```python
from build123d import *

# Parameters (mm, degrees)
RESSALTO_EXTRUS_O2_DEPTH = 9.2
ESBO_O5_R                = 2.15
CORTE_EXTRUS_O2_DEPTH    = 9.2
CHANFRO2_SIZE            = 0.3
SKETCH1_W                = 12.014068267
SKETCH1_H                = 17.223276929
CUT_EXTRUDE1_DEPTH       = 25
SKETCH3_W                = 4
SKETCH3_H                = 9.2
BOSS_EXTRUDE1_DEPTH      = 5
SKETCH4_R                = 1.5
CUT_EXTRUDE3_DEPTH       = 10
SKETCH5_W                = 42.60578415
SKETCH5_H                = 33.509789151
CUT_EXTRUDE4_DEPTH       = 1.1
SKETCH6_W                = 58.176505701
SKETCH6_H                = 25.888094607
CUT_EXTRUDE5_DEPTH       = 1.1
SKETCH7_W                = 20
SKETCH7_H                = 4.9
BOSS_EXTRUDE2_DEPTH      = 1.1
SKETCH8_W                = 20
SKETCH8_H                = 4.9
BOSS_EXTRUDE3_DEPTH      = 1.1


with BuildPart() as part:
    # Esboço4 → Ressalto-extrusão2 (new body)
    with BuildSketch(Plane(origin=(0, 0, 0), x_dir=(1, 0, 0), z_dir=(0, 1, 0))):
        with BuildLine():
            Line((-19.2, 2.35), (-19.2, 1.65))
            ThreePointArc((-19.2, 1.65), (-19.170710678, 1.579289322), (-19.1, 1.55))
            Line((-19.1, 1.55), (-18.1, 1.55))
            ThreePointArc((-18.1, 1.55), (-18.029289322, 1.579289322), (-18, 1.65))
            Line((-18, 1.65), (-18, 2.35))
            ThreePointArc((-18, 2.35), (-17.970710678, 2.420710678), (-17.9, 2.45))
            Line((-17.9, 2.45), (-17.3, 2.45))
            ThreePointArc((-17.3, 2.45), (-17.229289322, 2.420710678), (-17.2, 2.35))
            Line((-17.2, 2.35), (-17.2, 1.65))
            ThreePointArc((-17.2, 1.65), (-17.170710678, 1.579289322), (-17.1, 1.55))
            Line((-17.1, 1.55), (-16.1, 1.55))
            ThreePointArc((-16.1, 1.55), (-16.029289322, 1.579289322), (-16, 1.65))
            Line((-16, 1.65), (-16, 2.35))
            ThreePointArc((-16, 2.35), (-15.970710678, 2.420710678), (-15.9, 2.45))
            Line((-15.9, 2.45), (-15.3, 2.45))
            ThreePointArc((-15.3, 2.45), (-15.229289322, 2.420710678), (-15.2, 2.35))
            Line((-15.2, 2.35), (-15.2, 1.65))
            ThreePointArc((-15.2, 1.65), (-15.170710678, 1.579289322), (-15.1, 1.55))
            Line((-15.1, 1.55), (-14.1, 1.55))
            ThreePointArc((-14.1, 1.55), (-14.029289322, 1.579289322), (-14, 1.65))
            Line((-14, 1.65), (-14, 2.35))
            ThreePointArc((-14, 2.35), (-13.970710678, 2.420710678), (-13.9, 2.45))
            Line((-13.9, 2.45), (-13.3, 2.45))
            ThreePointArc((-13.3, 2.45), (-13.229289322, 2.420710678), (-13.2, 2.35))
            Line((-13.2, 2.35), (-13.2, 1.65))
            ThreePointArc((-13.2, 1.65), (-13.170710678, 1.579289322), (-13.1, 1.55))
            Line((-13.1, 1.55), (-12.1, 1.55))
            ThreePointArc((-12.1, 1.55), (-12.029289322, 1.579289322), (-12, 1.65))
            Line((-12, 1.65), (-12, 2.35))
            ThreePointArc((-12, 2.35), (-11.970710678, 2.420710678), (-11.9, 2.45))
            Line((-11.9, 2.45), (-11.3, 2.45))
            ThreePointArc((-11.3, 2.45), (-11.229289322, 2.420710678), (-11.2, 2.35))
            Line((-11.2, 2.35), (-11.2, 1.65))
            ThreePointArc((-11.2, 1.65), (-11.170710678, 1.579289322), (-11.1, 1.55))
            Line((-11.1, 1.55), (-10.1, 1.55))
            ThreePointArc((-10.1, 1.55), (-10.029289322, 1.579289322), (-10, 1.65))
            Line((-10, 1.65), (-10, 2.35))
            ThreePointArc((-10, 2.35), (-9.970710678, 2.420710678), (-9.9, 2.45))
            Line((-9.9, 2.45), (-9.3, 2.45))
            ThreePointArc((-9.3, 2.45), (-9.229289322, 2.420710678), (-9.2, 2.35))
            Line((-9.2, 2.35), (-9.2, 1.65))
            ThreePointArc((-9.2, 1.65), (-9.170710678, 1.579289322), (-9.1, 1.55))
            Line((-9.1, 1.55), (-8.1, 1.55))
            ThreePointArc((-8.1, 1.55), (-8.029289322, 1.579289322), (-8, 1.65))
            Line((-8, 1.65), (-8, 2.35))
            ThreePointArc((-8, 2.35), (-7.970710678, 2.420710678), (-7.9, 2.45))
            Line((-7.9, 2.45), (-7.3, 2.45))
            ThreePointArc((-7.3, 2.45), (-7.229289322, 2.420710678), (-7.2, 2.35))
            Line((-7.2, 2.35), (-7.2, 1.65))
            ThreePointArc((-7.2, 1.65), (-7.170710678, 1.579289322), (-7.1, 1.55))
            Line((-7.1, 1.55), (7.1, 1.55))
            ThreePointArc((7.1, 1.55), (7.170710678, 1.579289322), (7.2, 1.65))
            Line((7.2, 1.65), (7.2, 2.35))
            ThreePointArc((7.2, 2.35), (7.229289322, 2.420710678), (7.3, 2.45))
            Line((7.3, 2.45), (7.9, 2.45))
            ThreePointArc((7.9, 2.45), (7.970710678, 2.420710678), (8, 2.35))
            Line((8, 2.35), (8, 1.65))
            ThreePointArc((8, 1.65), (8.029289322, 1.579289322), (8.1, 1.55))
            Line((8.1, 1.55), (9.1, 1.55))
            ThreePointArc((9.1, 1.55), (9.170710678, 1.579289322), (9.2, 1.65))
            Line((9.2, 1.65), (9.2, 2.35))
            ThreePointArc((9.2, 2.35), (9.229289322, 2.420710678), (9.3, 2.45))
            Line((9.3, 2.45), (9.9, 2.45))
            ThreePointArc((9.9, 2.45), (9.970710678, 2.420710678), (10, 2.35))
            Line((10, 2.35), (10, 1.65))
            ThreePointArc((10, 1.65), (10.029289322, 1.579289322), (10.1, 1.55))
            Line((10.1, 1.55), (11.1, 1.55))
            ThreePointArc((11.1, 1.55), (11.170710678, 1.579289322), (11.2, 1.65))
            Line((11.2, 1.65), (11.2, 2.35))
            ThreePointArc((11.2, 2.35), (11.229289322, 2.420710678), (11.3, 2.45))
            Line((11.3, 2.45), (11.9, 2.45))
            ThreePointArc((11.9, 2.45), (11.970710678, 2.420710678), (12, 2.35))
            Line((12, 2.35), (12, 1.65))
            ThreePointArc((12, 1.65), (12.029289322, 1.579289322), (12.1, 1.55))
            Line((12.1, 1.55), (13.1, 1.55))
            ThreePointArc((13.1, 1.55), (13.170710678, 1.579289322), (13.2, 1.65))
            Line((13.2, 1.65), (13.2, 2.35))
            ThreePointArc((13.2, 2.35), (13.229289322, 2.420710678), (13.3, 2.45))
            Line((13.3, 2.45), (13.9, 2.45))
            ThreePointArc((13.9, 2.45), (13.970710678, 2.420710678), (14, 2.35))
            Line((14, 2.35), (14, 1.65))
            ThreePointArc((14, 1.65), (14.029289322, 1.579289322), (14.1, 1.55))
            Line((14.1, 1.55), (15.1, 1.55))
            ThreePointArc((15.1, 1.55), (15.170710678, 1.579289322), (15.2, 1.65))
            Line((15.2, 1.65), (15.2, 2.35))
            ThreePointArc((15.2, 2.35), (15.229289322, 2.420710678), (15.3, 2.45))
            Line((15.3, 2.45), (15.9, 2.45))
            ThreePointArc((15.9, 2.45), (15.970710678, 2.420710678), (16, 2.35))
            Line((16, 2.35), (16, 1.65))
            ThreePointArc((16, 1.65), (16.029289322, 1.579289322), (16.1, 1.55))
            Line((16.1, 1.55), (17.1, 1.55))
            ThreePointArc((17.1, 1.55), (17.170710678, 1.579289322), (17.2, 1.65))
            Line((17.2, 1.65), (17.2, 2.35))
            ThreePointArc((17.2, 2.35), (17.229289322, 2.420710678), (17.3, 2.45))
            Line((17.3, 2.45), (17.9, 2.45))
            ThreePointArc((17.9, 2.45), (17.970710678, 2.420710678), (18, 2.35))
            Line((18, 2.35), (18, 1.65))
            ThreePointArc((18, 1.65), (18.029289322, 1.579289322), (18.1, 1.55))
            Line((18.1, 1.55), (19.1, 1.55))
            ThreePointArc((19.1, 1.55), (19.170710678, 1.579289322), (19.2, 1.65))
            Line((19.2, 1.65), (19.2, 2.35))
            ThreePointArc((19.2, 2.35), (19.229289322, 2.420710678), (19.3, 2.45))
            Line((19.3, 2.45), (19.9, 2.45))
            ThreePointArc((19.9, 2.45), (19.970710678, 2.420710678), (20, 2.35))
            Line((20, 2.35), (20, -2.45))
            Line((20, -2.45), (-20, -2.45))
            Line((-20, -2.45), (-20, 2.35))
            ThreePointArc((-20, 2.35), (-19.970710678, 2.420710678), (-19.9, 2.45))
            Line((-19.9, 2.45), (-19.3, 2.45))
            ThreePointArc((-19.3, 2.45), (-19.229289322, 2.420710678), (-19.2, 2.35))
        make_face()
    extrude(amount=RESSALTO_EXTRUS_O2_DEPTH)

    # Esboço5 → Corte-extrusão2 (cut)
    with BuildSketch(Plane(origin=(0, 0, -1.55), x_dir=(-1, 0, 0), z_dir=(0, 0, -1))):
        with Locations((0, 4.6)):
            Circle(ESBO_O5_R)
    extrude(amount=-CORTE_EXTRUS_O2_DEPTH, mode=Mode.SUBTRACT)

    # Chanfro2
    chanfro2_edges = [part.edges().sort_by_distance(p)[0] for p in [
        (2.15, 4.6, -1.55),
    ]]
    chamfer(chanfro2_edges, length=CHANFRO2_SIZE)

    # Sketch1 → Cut-Extrude1 (cut)
    with BuildSketch(Plane(origin=(20, 0, 0), x_dir=(0, 0, -1), z_dir=(1, 0, 0))):
        with Locations((-0.254525551, 3.53223116)):
            Rectangle(SKETCH1_W, SKETCH1_H)
    extrude(amount=-CUT_EXTRUDE1_DEPTH, mode=Mode.SUBTRACT)

    # Sketch3 → Boss-Extrude1 (add)
    with BuildSketch(Plane(origin=(-5, 0, 0), x_dir=(0, 0, -1), z_dir=(1, 0, 0))):
        with Locations((-0.45, 4.6)):
            Rectangle(SKETCH3_W, SKETCH3_H)
    extrude(amount=BOSS_EXTRUDE1_DEPTH)

    # Sketch4 → Cut-Extrude3 (cut)
    with BuildSketch(Plane(origin=(0, 0, -1.55), x_dir=(-1, 0, 0), z_dir=(0, 0, -1))):
        with Locations((5, 4.6)):
            Circle(SKETCH4_R)
    extrude(amount=-CUT_EXTRUDE3_DEPTH, mode=Mode.SUBTRACT)

    # Sketch5 → Cut-Extrude4 (cut)
    with BuildSketch(Plane.XZ):
        with Locations((-12.27909741, -6.492410197)):
            Rectangle(SKETCH5_W, SKETCH5_H)
    extrude(amount=-CUT_EXTRUDE4_DEPTH, mode=Mode.SUBTRACT)

    # Sketch6 → Cut-Extrude5 (cut)
    with BuildSketch(Plane(origin=(0, 9.2, 0), x_dir=(1, 0, 0), z_dir=(0, 1, 0))):
        with Locations((-5.279993837, 3.701095613)):
            Rectangle(SKETCH6_W, SKETCH6_H)
    extrude(amount=-CUT_EXTRUDE5_DEPTH, mode=Mode.SUBTRACT)

    # Sketch7 → Boss-Extrude2 (add)
    with BuildSketch(Plane(origin=(0, 8.1, 0), x_dir=(1, 0, 0), z_dir=(0, 1, 0))):
        with Locations((-10, 0)):
            Rectangle(SKETCH7_W, SKETCH7_H)
    extrude(amount=BOSS_EXTRUDE2_DEPTH)

    # Sketch8 → Boss-Extrude3 (add)
    with BuildSketch(Plane.XZ.offset(-1.1)):
        with Locations((-10, 0)):
            Rectangle(SKETCH8_W, SKETCH8_H)
    extrude(amount=BOSS_EXTRUDE3_DEPTH)


solid = part.part
```
Model file for the job. Use its own axes, mm. A direction names the side the tool comes from. Give positions to 0.01 mm unless a question says otherwise; leave off trailing zeros. Loops run counter-clockwise (first coordinate to the right, second up) from the corner with the lowest first, then second, coordinate; pieces in that order, holes last. Notation, with made-up numbers: (-31.5, 43.25) - (-24.5, 43.25) arc R23 cw to (-24.5, 57.25) - close; hole circle Ø2 at (31.25, 47). An arc over 180 degrees is marked (long way). One line per item, written item: value. Start each with the question number.
1. Pin check, flat tips, straight feed: pin 1 (3.5 mm diameter, centred on x = -5, y = 6, fed in from -Z); pin 2 (1.1 mm diameter, centred on x = -15, y = 3.5, fed in from -Z). Stop position of each tip, or through.
2. Slice it at C-C (z = 0.3). List the corners of the cut face in (x, y).
3. Pull direction Y, two halves, no side cores. Call faces 1 (the flat face through (-15, 8.1, -2)), 2 (the flat face through (-10, 9.2, 0)), 3 (the flat face through (0, 5, 1)): pulls with the +Y half, pulls with the -Y half, needs draft (parallel to the pull), parting line crosses it, or undercut.
4. Slice it at A-A (x = -5). List the corners of the cut face in (y, z), plus the area to 3 significant figures.
5. Slice it at B-B (z = -2). Give the number of separate pieces and of enclosed holes in the cut face, plus the area to 3 significant figures.
6. Probe L1, parallel to Y at x = -5, z = -0.4; L2, parallel to Y at x = -16.75, z = -2.15; L3, parallel to Z at x = -1.75, y = 7. List the from-to ranges inside material, lowest first. Write a range as from..to.
7. Which spindle directions (+Z, -Z, +X, -X, +Y, -Y) get a long thin tool onto all of the face, cutting with end or side? Do faces 4 (the flat face through (-11, 8.1, -2)), 5 (the flat face through (-4, 1.1, -2)), 6 (the flat face through (-20, 5, 0)). Say none if no direction does.
8. Slice it at D-D (x = -3). List the corners of the cut face in (y, z).
Solution:
1. pin 1: stops at z = -1.55
1. pin 2: stops at z = -2.45
2. outline: (-20, 0) - (0, 0) - (0, 9.2) - (-20, 9.2) - close; hole circle Ø3 at (-5, 4.6)
3. face 1: undercut
3. face 2: pulls with the +Y half
3. face 3: needs draft
4. outline: (0, -2.45) - (1.1, -2.45) - (1.1, -1.55) - (3.1, -1.55) - (3.1, 2.45) - (0, 2.45) - close; (6.1, -1.55) - (8.1, -1.55) - (8.1, -2.45) - (9.2, -2.45) - (9.2, 2.45) - (6.1, 2.45) - close
4. area: 26.8 mm^2
5. separate pieces: 1
5. enclosed holes: 6
5. area: 83.2 mm^2
6. L1: y = 0..3.1, 6.1..9.2
6. L2: y = 0..1.1, 8.1..9.2
6. L3: z = -1.55..2.45
7. face 4: -Z
7. face 5: -Z, +X
7. face 6: +Z, -Z, -X, +Y, -Y
8. outline: (0, -2.45) - (1.1, -2.45) - (1.1, -1.55) - (8.1, -1.55) - (8.1, -2.45) - (9.2, -2.45) - (9.2, 2.45) - (0, 2.45) - close
